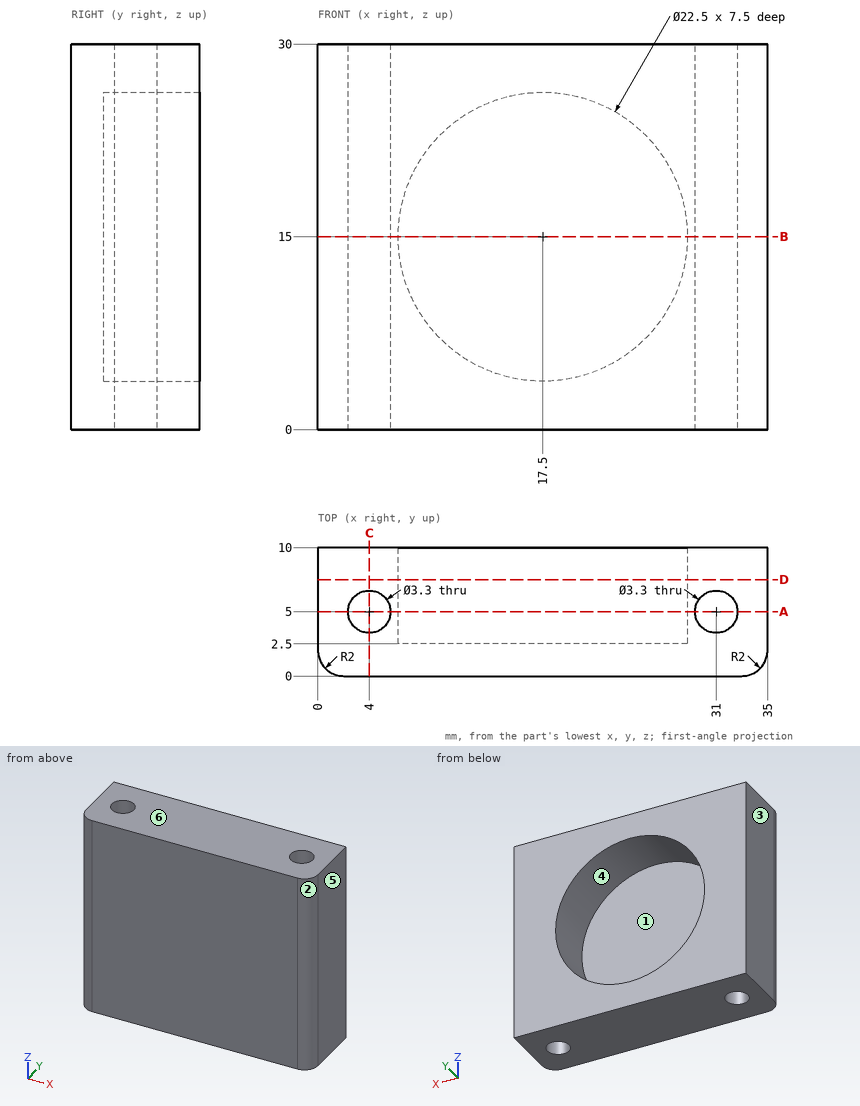
Study the drawing (mm; zero at the part's minimum x, y, z) and answer. A direction names the side the tool comes from. Round coordinates to 2 decimals unless told otherwise and drop trailing zeros. Write each loop counter-clockwise with the first axis right and the second up, starting at its lowest first coordinate (ties: lowest second). Pieces come first, ordered by that corner, then holes. Notation, with made-up numbers: (23, -25) -> (73, -25) arc R33 ccw to (73, 3) -> close; hole circle Ø8 at (11.25, 3.5). An arc over 180 degrees is marked (long way). Write item = value, one per line.
1) Section C-C on x = 4 is taken. Write down the section's boundary in (y, z).
Check values:
outline = (0, 0) -> (3.35, 0) -> (3.35, 30) -> (0, 30) -> close; (6.65, 0) -> (10, 0) -> (10, 30) -> (6.65, 30) -> close
2) Given pin 1 (2 mm diameter, centred on x = 27.5, z = 17, fed in from +Y); pin 2 (2.5 mm diameter, centred on x = 31, y = 5, fed in from -Z), each flat-ended and moving along its own axis, determine where each tip first touches the part or whether it passes through.
Check values:
pin_1 = 2.5
pin_2 = through
3) Section B-B on z = 15 is taken. Write down the section's boundary in (x, y), plus the area to 3 significant figures.
Check values:
outline = (0, 2) arc R2 ccw to (2, 0) -> (33, 0) arc R2 ccw to (35, 2) -> (35, 10) -> (28.75, 10) -> (28.75, 2.5) -> (6.25, 2.5) -> (6.25, 10) -> (0, 10) -> close; hole circle Ø3.3 at (4, 5); hole circle Ø3.3 at (31, 5)
area = 162 mm²
4) For a pull along X with two mould halves and no side action, classify the marked faces 3, 4, 5 and 6 as released by +X, released by -X, zero draft, split by the parting line, or undercut.
Check values:
face_3 = released by -X
face_4 = undercut
face_5 = released by +X
face_6 = zero draft
5) Which of the six approach directions +Z, -Z, +X, -X, +Y, -Y give full straight-line access (tool end or side, diameter ignored) to the marked faces 1 and 2?
Check values:
face_1 = +Y
face_2 = +Z, -Z, +X, -Y
6) Section D-D on y = 7.5 is taken. Write down the section's boundary in (x, z).
Check values:
outline = (0, 0) -> (35, 0) -> (35, 30) -> (0, 30) -> close; hole circle Ø22.5 at (17.5, 15)
7) Section A-A on y = 5 is taken. Write down the section's boundary in (x, z), plus the area to 3 significant figures.
Check values:
outline = (0, 0) -> (2.35, 0) -> (2.35, 30) -> (0, 30) -> close; (5.65, 0) -> (29.35, 0) -> (29.35, 30) -> (5.65, 30) -> close; (32.65, 0) -> (35, 0) -> (35, 30) -> (32.65, 30) -> close; hole circle Ø22.5 at (17.5, 15)
area = 454 mm²
8) Straight lines are drawn through the part: line 1 along Z through (x, y) = (17.5, 6); line 2 along Y through (x, z) = (4, 6.75); line 3 along X through (y, z) = (6.5, 15). For each, find the intervals that lie inside material, in ascending order. Write a range as [from, to].
Check values:
line_1 = [0, 3.75], [26.25, 30]
line_2 = [0, 3.35], [6.65, 10]
line_3 = [0, 3.31], [4.69, 6.25], [28.75, 30.31], [31.69, 35]
